Can you work these out from the model? Positions are in its coordinate system, mm. A direction names the side the tool comes from. Round coordinates to 2 decimals unless told otherwise and drop trailing zeros. Write each loop counter-clockwise with the first axis right and the second up, starting at its lowest first coordinate (ties: lowest second). Pieces come first, ordered by that corner, then holes. Notation, with made-up numbers: M -21,25.25 L 5,25.25 A15 cw 5,37.25 Z; hole C 74,-24 d8. An arc over 180 degrees is marked long. Use one line per item in the form item = value. Start each with the question number.
Autodesk Fusion 360 part; units mm, degrees
sketch "Sketch1" plane through (0, 0, 0) normal (1, 0, 0) x (0, 0, -1)
  line L0 (-16.6875, 45) -> (0, 45)
  line L1 (0, 45) -> (0, 0)
  line L2 (0, 0) -> (-16.6875, 0)
  arc A0 (-16.6875, 45) -> (-16.6875, 0) centre (-16.6875, 22.5) ccw
  circle A1 centre (-16.6875, 22.5) radius 11.125
  line L3 (0, 22.5) -> (-29, 22.5) construction
  circle A2 centre (-16.6875, 22.5) radius 9.125
  dimension "d1" = 22.25
  dimension "d2" = 45
  dimension "d3" = 16.6875
  dimension "d4" = -2
extrude "Extrude2" add sketch "Sketch1" along normal blind 10 contours L0 L1 L2 A0
sketch "Sketch2" plane through (0, 0, 0) normal (0, 0, -1) x (-1, 0, 0)
  line L0 (0, 45) -> (-10, 45)
  line L1 (-10, 0) -> (0, 0)
  circle A0 centre (-5, 5.2) radius 3.5
  line L2 (-5, 0) -> (-5, 4) construction
  circle A1 centre (-5, 5.2) radius 1.6
  line L3 (0, 0) -> (0, 45)
  line L4 (-10, 45) -> (-10, 0)
  dimension "d13" = 7
  dimension "d14" = 5.2
  dimension "d17" = 3.2
extrude "Extrude4" cut sketch "Sketch2" against normal blind 40 contours A0 | A1
extrude "Extrude5" add sketch "Sketch2" against normal blind 25.5 contours A0
ref_plane "WorkPlane1" through (5, 22.5, 8.3438) normal (0, -1, 0) x (0, 0, -1)
mirror "Mirror1" about plane through (5, 22.5, 8.3438) normal (0, -1, 0) of "Extrude4", "Extrude5"
equation "d3 = d1 * 0.75"
equation "d14 = d13 / 2 + 1.7 mm"
1. If we section it at B-B (z = 9.5): List the corners of the cut face in (x, y) for me, and give its area (3 significant figures).
2. If we section it at C-C (y = 22.5): List the corners of the cut face in (x, z) for me.
3. Will these pins go through, and if not, where does the flat tip stop? pin 1 (2 mm diameter, centred on x = 4, z = 34, fed in from -Y); pin 2 (20 mm diameter, centred on y = 22.5, z = 16.69, fed in from -X); pin 3 (1 mm diameter, centred on x = 7.5, z = 18, fed in from +Y); pin 4 (1 mm diameter, centred on x = 4.5, z = 23, fed in from -Y).
4. If we mould it in two halves opening along Y, with no side actions, what happens to faces 1 (the face through (5, 45, 8)), 2 (the face through (10, 23, 29)), 3 (the face through (4.9, 8.7, 28.9)), 4 (the face through (6.18, 6.28, 12.57))? For each: pulls with the +Y half, pulls with the -Y half, needs draft (parallel to the pull), parting line crosses it, or undercut.
5. Which directions (+Z, -Z, +X, -X, +Y, -Y) give clear straight access to the entire face, cutting with the end or side of a thin tool? Please do faces 5 (the face through (4.93, 26.76, 6.41)), 6 (the face through (7, 41, 25.5)).
6. Please list where these lines run through material, in increasing order: line 1 along X through (y, z) = (5, 17); line 2 along Z through (x, y) = (0.5, 22); line 3 along Y through (x, z) = (2.75, 17).
7. If we section it at A-A (x = 5): State how many separate pieces and enclosed holes the cut face has, and give its area (3 significant figures).
Model answer:
q1.outline = M 0,0 L 10,0 L 10,14.01 L 0,14.01 Z; M 0,30.99 L 10,30.99 L 10,45 L 0,45 Z; hole C 5,5.2 d3.2; hole C 5,39.8 d3.2
q1.area = 264 mm2
q2.outline = M 0,0 L 10,0 L 10,5.56 L 0,5.56 Z; M 0,27.81 L 10,27.81 L 10,39.19 L 0,39.19 Z
q3.pin_1 = 8.07
q3.pin_2 = through
q3.pin_3 = 44.99
q3.pin_4 = 0.76
q4.face_1 = pulls with the +Y half
q4.face_2 = needs draft
q4.face_3 = undercut
q4.face_4 = undercut
q5.face_5 = +X, -X
q5.face_6 = +Z
q6.line_1 = 0 to 3.41, 6.59 to 10
q6.line_2 = 0 to 5.57, 27.8 to 39.18
q6.line_3 = 0 to 11.38, 33.62 to 45
q7.separate_pieces = 3
q7.enclosed_holes = 1
q7.area = 921 mm2
